from build123d import *

# Parameters (mm, degrees)
SKETCH1_W               = 152.4
SKETCH1_H               = 25.4
BOSS_EXTRUDE1_DEPTH     = 4.826
SKETCH2_W               = 38.1
SKETCH2_H               = 4.826
BOTTOM_EDGE_SLOTS_DEPTH = 155.577521898
SKETCH4_W               = 66.675
SKETCH4_H               = 4.826
TOP_EDGE_SLOT_DEPTH     = 155.577521898
SKETCH6_W               = 4.826
SKETCH6_H               = 15.748
LEADING_EDGE_CUT_DEPTH  = 155.577521898


with BuildPart() as part:
    # Sketch1 → Boss-Extrude1 (new body)
    with BuildSketch(Plane(origin=(0, 0, 0), x_dir=(0, 0, -1), z_dir=(1, 0, 0))):
        with Locations((76.2, 12.7)):
            Rectangle(SKETCH1_W, SKETCH1_H)
    extrude(amount=BOSS_EXTRUDE1_DEPTH)

    # Sketch2 → Bottom Edge Slots (cut, through all)
    with BuildSketch(Plane(origin=(4.826, 0, 0), x_dir=(0, 0, -1), z_dir=(1, 0, 0))):
        with Locations((19.05, 2.413)):
            Rectangle(SKETCH2_W, SKETCH2_H)
        with Locations((76.2, 2.413)):
            Rectangle(SKETCH2_W, SKETCH2_H)
        with Locations((133.35, 2.413)):
            Rectangle(SKETCH2_W, SKETCH2_H)
    extrude(amount=-BOTTOM_EDGE_SLOTS_DEPTH, mode=Mode.SUBTRACT)

    # Sketch4 → Top Edge Slot (cut, through all)
    with BuildSketch(Plane(origin=(4.826, 0, 0), x_dir=(0, 0, -1), z_dir=(1, 0, 0))):
        with Locations((33.3375, 22.987)):
            Rectangle(SKETCH4_W, SKETCH4_H)
        with Locations((119.0625, 22.987)):
            Rectangle(SKETCH4_W, SKETCH4_H)
    extrude(amount=-TOP_EDGE_SLOT_DEPTH, mode=Mode.SUBTRACT)

    # Sketch6 → Leading Edge Cut (cut, through all)
    with BuildSketch(Plane(origin=(4.826, 0, 0), x_dir=(0, 0, -1), z_dir=(1, 0, 0))):
        with Locations((2.413, 12.7)):
            Rectangle(SKETCH6_W, SKETCH6_H)
    extrude(amount=-LEADING_EDGE_CUT_DEPTH, mode=Mode.SUBTRACT)


solid = part.part
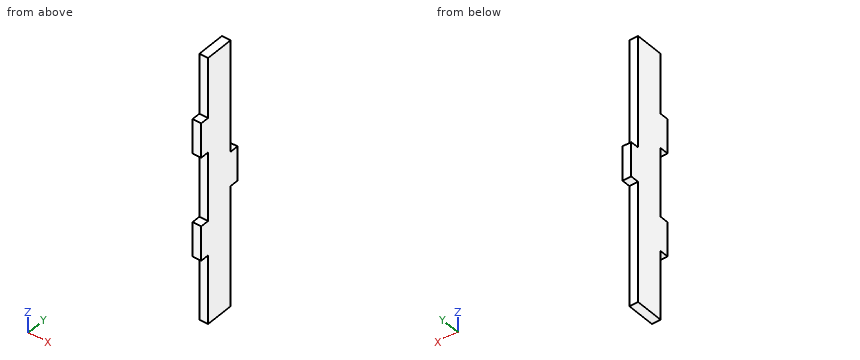
The model under review builds one solid part; all positions refer to its coordinate system, in mm. Give positions to 0.01 mm unless a question says otherwise; leave off trailing zeros. Order: outer loops, then holes, each group sorted by start corner. A loop starts at its lowest first (then second) coordinate and runs counter-clockwise, first axis right, second up. Notation, with made-up numbers: M 70.5,45.5 L 99.5,45.5 A18 ccw 99.5,53.5 Z; hole C 84,-18 d7. An arc over 180 degrees is marked long. Answer in a Markdown table with one row per item. Add a question column.
1. Add section B-B on z = -83. State the section outline as (x, y) points.
2. To check wall thickness, follow line 1 along Z through (x, y) = (1.55, 3.25); line 2 along Y through (x, z) = (3.15, -73); line 3 along Y through (x, z) = (0.3, -136.5). State the ranges of each line that lie inside material, in increasing order.
3. Add section A-A on x = 2.35. State the section outline as (y, z) points (3 decimals), plus the area to 3 significant figures.
4. For pin 1 Ø1.4 at (x, z) = (3.5, -14.5) entering from -Y; pin 2 Ø5 at (y, z) = (22.5, -37) entering from +X; pin 3 Ø2.5 at (x, z) = (1.5, -121) entering from +Y; pin 4 Ø2.5 at (x, y) = (2, 22) entering from +Z (3 decimals), all flat-tipped, find the tip position at first contact; note any pin that passes through.
5. Add section C-C on y = 23.25. State the section outline as (x, z) points (3 decimals).
The answers:
| question | item | result |
|---|---|---|
| 1 | outline | M 0,4.83 L 4.83,4.83 L 4.83,25.4 L 0,25.4 Z |
| 2 | line 1 | -114.3 to -95.25, -57.15 to -38.1 |
| 2 | line 2 | 4.83 to 25.4 |
| 2 | line 3 | 4.83 to 20.57 |
| 3 | outline | M 0,-114.3 L 4.826,-114.3 L 4.826,-152.4 L 20.574,-152.4 L 20.574,-85.725 L 25.4,-85.725 L 25.4,-66.675 L 20.574,-66.675 L 20.574,-4.826 L 4.826,-4.826 L 4.826,-38.1 L 0,-38.1 L 0,-57.15 L 4.826,-57.15 L 4.826,-95.25 L 0,-95.25 Z |
| 3 | area | 2,600 mm2 |
| 4 | pin 1 | y = 4.83 |
| 4 | pin 2 | x = 4.83 |
| 4 | pin 3 | y = 20.57 |
| 4 | pin 4 | z = -66.675 |
| 5 | outline | M 0,-85.725 L 4.826,-85.725 L 4.826,-66.675 L 0,-66.675 Z |
